Geometry: final body of the model. Coordinates: model frame, mm. Coordinates: 2 decimals unless noted, no trailing zeros. Write each loop counter-clockwise with the first axis right and the second up, starting at its lowest first coordinate (ties: lowest second). Pieces come first, ordered by that corner, then holes. Notation, with made-up numbers: (45, 48) -> (49, 48) arc R22 cw to (49, 77) -> close; hole circle Ø1 at (-28, 66). An arc over 180 degrees is marked (long way). Answer as a JSON object with one key per item and string values. Group by question number.
```python
from build123d import *

# Parameters (mm, degrees)
SKETCH1_W               = 1100
SKETCH1_H               = 1060
BOSS_EXTRUDE1_DEPTH     = 40
CUT_EXTRUDE1_DEPTH      = 1529.136119591
CUT_EXTRUDE1_DEPTH_BACK = 40


with BuildPart() as part:
    # Sketch1 → Boss-Extrude1 (new body)
    with BuildSketch(Plane.XY):
        with Locations((-550, 530)):
            Rectangle(SKETCH1_W, SKETCH1_H)
    extrude(amount=BOSS_EXTRUDE1_DEPTH)

    # Sketch2 → Cut-Extrude1 (cut, two sides: drawn at the far end of the back side and taken through both)
    with BuildSketch(Plane.XY.offset(40).offset(-CUT_EXTRUDE1_DEPTH_BACK)):
        Polygon((-2197.89099578, 2957.89099578), (-300, 1060), (0, 760), (1897.89099578, -1137.89099578), (5693.672987339, 2657.89099578), (1597.89099578, 6753.672987339), align=None)
    extrude(amount=CUT_EXTRUDE1_DEPTH + CUT_EXTRUDE1_DEPTH_BACK, mode=Mode.SUBTRACT)


solid = part.part
```
Item 1: Section A-A on z = 19. Output: boundary loops of the cut face in (x, y).
Item 2: Section B-B on y = 829. Output: boundary loops of the cut face in (x, z).
Item 3: Contact query for a flat-ended pin moving along its axis: pin 1 (4 mm diameter, centred on x = -269.5, z = 33.5, fed in from +Y). Output: stop coordinate, or through.
Item 4: Section C-C on x = -265. Output: boundary loops of the cut face in (y, z).
Item 5: Ray query, L1, parallel to Y at x = -262.5, z = 11.5; L2, parallel to Y at x = -154, z = 6. Return the intervals inside material, ascending. Write a range as [from, to].
Answer sheet:
{
 "1": {"outline": "(-1100, 0) -> (0, 0) -> (0, 760) -> (-300, 1060) -> (-1100, 1060) -> close"},
 "2": {"outline": "(-1100, 0) -> (-69, 0) -> (-69, 40) -> (-1100, 40) -> close"},
 "3": {"pin 1": "stops at y = 1031.5"},
 "4": {"outline": "(0, 0) -> (1025, 0) -> (1025, 40) -> (0, 40) -> close"},
 "5": {"L1": "y = [0, 1022.5]", "L2": "y = [0, 914]"}
}
